Design review of the part built by this model. Coordinates are the model's own, in mm. Face numbers are marked on the shaded views. A direction names the side the tool comes from. Coordinates: 2 decimals unless noted, no trailing zeros. Write each loop counter-clockwise with the first axis right and the second up, starting at its lowest first coordinate (ties: lowest second). Pieces come first, ordered by that corner, then holes. Notation, with made-up numbers: (-30.75, 62) - (-24.75, 62) arc R32 cw to (-24.75, 97) - close; hole circle Ø5 at (62.25, 84). An arc over 180 degrees is marked (long way). Answer as CSV lines item,"result". Start each with the question number.
Q1. Mouldability with a two-part tool opening along X and no side actions: class the marked faces 4, 5, 6 and 7 as pulls with the +X half, pulls with the -X half, needs draft (parallel to the pull), parting line crosses it, or undercut.
Q2. Clearance check with a flat-ended pin moving along its axis: pin 1 (3.5 mm diameter, centred on x = 7.88, y = 7.87, fed in from -Z). State where the tip first meets the part, or that it passes through.
Q3. We need section A-A (z = 7.5). Write out the cut boundary in (x, y).
Q4. We need section B-B (y = 7.87). Write out the cut boundary in (x, z), plus the area to 3 significant figures.
Q5. We need section C-C (x = 13.75). Write out the cut boundary in (y, z), plus the area to 3 significant figures.
Q6. For line 1 along X through (y, z) = (7.87, 3.5); line 2 along Y through (x, z) = (12.5, 1); line 3 along Y through (x, z) = (9.25, 6.5), list the stretches that pass through material, from the lowest coordinate up. Write a range as [from, to].
Q7. Machinability: for the marked faces 1, 2 and 3, which of the approach directions +Z, -Z, +X, -X, +Y, -Y give a long, thin tool a straight path to every point of the face, cutting with its end or side? Answer none if there is none.
from build123d import *

# Parameters (mm, degrees)
F0_W     = 15.74
F0_H     = 15.74
F1_DEPTH = 9.59
F3_DEPTH = 2
F4_R     = 2.57
F5_DEPTH = 8
F4_R_2   = 2.2615660893
F6_DEPTH = 8


with BuildPart() as f1:
    # F0 (on Top) → F1 (new body)
    with BuildSketch(Plane.XY):
        with Locations((7.87, 7.87)):
            Rectangle(F0_W, F0_H)
    extrude(amount=F1_DEPTH)

    # F2 (on face) → F3 (join)
    with BuildSketch(Plane.XY.offset(9.59)):
        with BuildLine():
            ThreePointArc((6.36, 11.805), (6.1754078663, 12.7330073235), (5.6497339444, 13.5197339444))
            Line((5.6497339444, 13.5197339444), (2.2202660556, 10.0902660556))
            ThreePointArc((2.2202660556, 10.0902660556), (4.8630073235, 9.5645921337), (6.36, 11.805))
        make_face()
        with BuildLine():
            Line((2.2202660556, 10.0902660556), (5.6497339444, 13.5197339444))
            ThreePointArc((5.6497339444, 13.5197339444), (2.2202660556, 13.5197339444), (2.2202660556, 10.0902660556))
        make_face()
        with BuildLine():
            ThreePointArc((14.23, 11.805), (12.7330073235, 14.0454078663), (10.0902660556, 13.5197339444))
            Line((10.0902660556, 13.5197339444), (13.5197339444, 10.0902660556))
            ThreePointArc((13.5197339444, 10.0902660556), (14.0454078663, 10.8769926765), (14.23, 11.805))
        make_face()
        with BuildLine():
            Line((13.5197339444, 10.0902660556), (10.0902660556, 13.5197339444))
            ThreePointArc((10.0902660556, 13.5197339444), (10.0902660556, 10.0902660556), (13.5197339444, 10.0902660556))
        make_face()
        with BuildLine():
            Line((13.5197339444, 5.6497339444), (10.0902660556, 2.2202660556))
            ThreePointArc((10.0902660556, 2.2202660556), (12.7330073235, 1.6945921337), (14.23, 3.935))
            ThreePointArc((14.23, 3.935), (14.0454078663, 4.8630073235), (13.5197339444, 5.6497339444))
        make_face()
        with BuildLine():
            ThreePointArc((13.5197339444, 5.6497339444), (10.0902660556, 5.6497339444), (10.0902660556, 2.2202660556))
            Line((10.0902660556, 2.2202660556), (13.5197339444, 5.6497339444))
        make_face()
        with BuildLine():
            Line((2.2202660556, 5.6497339444), (5.6497339444, 2.2202660556))
            ThreePointArc((5.6497339444, 2.2202660556), (6.1754078663, 3.0069926765), (6.36, 3.935))
            ThreePointArc((6.36, 3.935), (4.8630073235, 6.1754078663), (2.2202660556, 5.6497339444))
        make_face()
        with BuildLine():
            ThreePointArc((2.2202660556, 5.6497339444), (2.2202660556, 2.2202660556), (5.6497339444, 2.2202660556))
            Line((5.6497339444, 2.2202660556), (2.2202660556, 5.6497339444))
        make_face()
    extrude(amount=F3_DEPTH)

    # F4 (on face) → F5 (cut)
    with BuildSketch(Plane(origin=(0, 0, 0), x_dir=(1, 0, 0), z_dir=(0, 0, -1))):
        Polygon((14.5437045489, -1.22), (1.22, -1.22), (1.22, -14.52), (14.4962799393, -14.52), align=None)
        with Locations((7.8818522745, -7.87)):
            Circle(F4_R, mode=Mode.SUBTRACT)
    extrude(amount=-F5_DEPTH, mode=Mode.SUBTRACT)

    # F4 (on face) → F6 (cut)
    with BuildSketch(Plane(origin=(0, 0, 0), x_dir=(1, 0, 0), z_dir=(0, 0, -1))):
        with Locations((7.8818522745, -7.87)):
            Circle(F4_R_2)
    extrude(amount=-F6_DEPTH, mode=Mode.SUBTRACT)


solid = f1.part
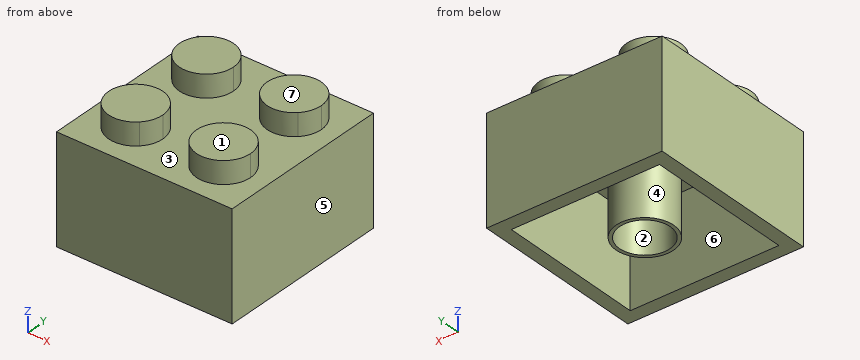
Results list:
1,face 4,"undercut"
1,face 5,"pulls with the +X half"
1,face 6,"undercut"
1,face 7,"needs draft"
2,pin 1,"stops at z = 8"
3,outline,"(0, 0) - (15.74, 0) - (15.74, 15.74) - (0, 15.74) - close; circle Ø5.14 at (7.88, 7.87); hole (1.22, 1.22) - (14.54, 1.22) - (14.5, 14.52) - (1.22, 14.52) - close; hole circle Ø4.52 at (7.88, 7.87)"
4,outline,"(0, 0) - (1.22, 0) - (1.22, 8) - (5.31, 8) - (5.31, 0) - (5.62, 0) - (5.62, 8) - (10.14, 8) - (10.14, 0) - (10.45, 0) - (10.45, 8) - (14.52, 8) - (14.52, 0) - (15.74, 0) - (15.74, 9.59) - (0, 9.59) - close"
4,area,"49.5 mm2"
5,outline,"(0, 0) - (1.22, 0) - (1.22, 8) - (14.52, 8) - (14.52, 0) - (15.74, 0) - (15.74, 9.59) - (13.25, 9.59) - (13.25, 11.59) - (10.36, 11.59) - (10.36, 9.59) - (5.38, 9.59) - (5.38, 11.59) - (2.49, 11.59) - (2.49, 9.59) - (0, 9.59) - close"
5,area,"56.1 mm2"
6,line 1,"x = [0, 1.22], [5.31, 5.62], [10.14, 10.45], [14.52, 15.74]"
6,line 2,"y = [0, 1.22], [14.52, 15.74]"
6,line 3,"y = [0, 1.22], [5.69, 6.07], [9.67, 10.05], [14.52, 15.74]"
7,face 1,"+Z, +X, -X, +Y, -Y"
7,face 2,"-Z"
7,face 3,"+Z"
